CAD build for the part. Positions are in the model's coordinates, mm. Give positions to 0.01 mm unless a question says otherwise; leave off trailing zeros.
from build123d import *

# Parameters (mm, degrees)
SKETCH1_W          = 50
SKETCH1_H          = 50
SKETCH2_W          = 100
SKETCH2_H          = 100
SKETCH3_R          = 5
SKETCH6_R          = 5
SKETCH7_R          = 7.5
CUT_EXTRUDE1_DEPTH = 101.0000001


with BuildPart() as part:
    # Sketch1 → Loft1 section 0
    with BuildSketch(Plane(origin=(0, 0, 0), x_dir=(0, 0, -1), z_dir=(1, 0, 0))):
        Rectangle(SKETCH1_W, SKETCH1_H)
    # Sketch2 → Loft1 section 1
    with BuildSketch(Plane(origin=(-100, 0, 0), x_dir=(0, 0, -1), z_dir=(1, 0, 0))):
        Rectangle(SKETCH2_W, SKETCH2_H)
    loft()

    # Cut-Sweep2: sweep along a path in Sketch4
    with BuildLine(Plane(origin=(0, 0, 0), x_dir=(1, 0, 0), z_dir=(0, 1, 0))) as cut_sweep2_path:
        Line((0, 15), (-100, 40))
    # Sketch3 → Cut-Sweep2 (sweep, cut)
    with BuildSketch(Plane(origin=(0, 0, 0), x_dir=(0, 0, -1), z_dir=(1, 0, 0))):
        with Locations((15, 0)):
            Circle(SKETCH3_R)
    cut_sweep2 = sweep(path=cut_sweep2_path.line, mode=Mode.SUBTRACT)

    # Cut-Sweep3: sweep along a path in Sketch5
    with BuildLine(Plane.XY) as cut_sweep3_path:
        Line((0, 15), (-100, 40))
    # Sketch6 → Cut-Sweep3 (sweep, cut)
    with BuildSketch(Plane(origin=(0, 0, 0), x_dir=(0, 0, -1), z_dir=(1, 0, 0))):
        with Locations((0, 15)):
            Circle(SKETCH6_R)
    cut_sweep3 = sweep(path=cut_sweep3_path.line, mode=Mode.SUBTRACT)

    # Mirror1: Cut-Sweep2 across plane
    add(cut_sweep2.mirror(Plane.XY), mode=Mode.SUBTRACT)

    # Mirror2: Cut-Sweep3 across plane
    add(cut_sweep3.mirror(Plane.ZX), mode=Mode.SUBTRACT)

    # Sketch7 → Cut-Extrude1 (cut, through all)
    with BuildSketch(Plane(origin=(0, 0, 0), x_dir=(0, 0, -1), z_dir=(1, 0, 0))):
        Circle(SKETCH7_R)
    extrude(amount=-CUT_EXTRUDE1_DEPTH, mode=Mode.SUBTRACT)


solid = part.part
1. Mould opens along Y. For faces 1 (the flat face through (0, 6, 6)), 2 (the cylindrical face through (-49.3, 0.33, 7.493)) say: released by +Y, released by -Y, zero draft, split by the parting line, or undercut.
2. Wall check: line 1 (Y direction, x = -69, z = 0); line 2 (Y direction, x = -75.5, z = 0) (3 decimals); line 3 (Z direction, x = -12.5, y = -4) (3 decimals). Give the ranges that are in metal, low to high.
3. Saw through at A-A on y = 0. State how many separate pieces and enclosed holes the cut face has, plus the area to 3 significant figures.
4. Pin check, flat tips, straight feed: P1, Ø2, axis at x = -48, z = 35, coming from the -Y side; P2, Ø5, axis at x = -39, z = -36, coming from the +Y side; P3, Ø6, axis at x = -19, z = -4.5, coming from the +Y side. Stop position of each tip, or through.
Reported:
1. face 1: zero draft
1. face 2: undercut
2. line 1: y = -42.25 to -37.25, -27.25 to -7.5, 7.5 to 27.25, 37.25 to 42.25
2. line 2: y = -43.875 to -38.875, -28.875 to -7.5, 7.5 to 28.875, 38.875 to 43.875
2. line 3: z = -28.125 to -21.125, -15.125 to -6.344, 6.344 to 15.125, 21.125 to 28.125
3. separate pieces: 4
3. enclosed holes: 0
3. area: 4,000 mm2
4. P1: stops at y = -37.25
4. P2: stops at y = 35.35
4. P3: stops at y = 30.5
